For this review, take the finished solid that the model builds, in its own axes (mm). A direction names the side the tool comes from. Coordinates: 2 decimals unless noted, no trailing zeros. Loops run counter-clockwise (first coordinate to the right, second up) from the corner with the lowest first, then second, coordinate; pieces in that order, holes last. Notation, with made-up numbers: (64, 75) - (116, 75) arc R28 ccw to (116, 110) - close; hole circle Ø2 at (45.25, -2). An arc over 180 degrees is marked (long way). Use one line per item in the form item = value. Start each with the question number.
1. Add section A-A on z = 2.8. Give the boundary of the cut face in (x, y), and give its area (3 significant figures).
2. Add section D-D on y = 42.75. Give the boundary of the cut face in (x, z), and give its area (3 significant figures).
3. To check wall thickness, follow probe 1 along X at (y, z) = (33, 0.1); probe 2 along X at (y, z) = (32.5, 2.55); probe 3 along X at (y, z) = (45.5, 1.45). State the ranges of each line that lie inside material, in increasing order.
4. Draft analysis for pull direction X (two halves, no side actions). For faces 1 (the face through (98.017, 29, 2)), 2 (the face through (81, 36.5, 3.25)), 3 (the face through (83.767, 34, 2)), state which applies: +X half, -X half, draft (parallel to the pull), parting line (faces both ways), or undercut.
5. Add section C-C on x = 95.5. Give the boundary of the cut face in (y, z).
6. For pin 1 Ø1 at (x, z) = (82, 1) entering from -Y; pin 2 Ø1 at (y, z) = (46, 2.5) entering from +X; pin 3 Ø1.6 at (y, z) = (24, 1.5) entering from -X, all flat-tipped, find the tip position at first contact; note any pin that passes through.
7. Machinability: for faces 4 (the face through (66, 27.022, 2)), 5 (the face through (94.767, 34, 2)), 6 (the face through (94.767, 25, 2)), 7 (the face through (67.767, 34, 2)), which of the approach directions +Z, -Z, +X, -X, +Y, -Y give a long, thin tool a straight path to every point of the face, cutting with its end or side? Answer none if there is none.
8. Add section B-B on y = 33.25. Give the boundary of the cut face in (x, z), and give its area (3 significant figures).
Autodesk Inventor part; units mm, degrees
ref_plane "YZ Plane" through (0, 0, 0) normal (1, 0, 0) x (0, 1, 0)
ref_plane "XZ Plane" through (0, 0, 0) normal (0, 1, 0) x (-1, 0, 0)
ref_plane "XY Plane" through (0, 0, 0) normal (0, 0, 1) x (1, 0, 0)
sketch "Block1" plane through (0, 0, 0) normal (0, 0, 1) x (1, 0, 0)
  circle A0 centre (74.029, 24.2723) radius 1
  line L0 (49.279, 30.4723) -> (71.779, 30.4723)
  line L1 (71.779, 30.4723) -> (71.779, 18.0723)
  line L2 (71.779, 18.0723) -> (49.279, 18.0723)
  line L3 (49.279, 18.0723) -> (49.279, 30.4723)
  line L4 (49.279, 30.4723) -> (44.779, 30.4723)
  line L5 (44.779, 30.4723) -> (44.779, 18.0723)
  line L6 (44.779, 18.0723) -> (49.279, 18.0723)
  line L7 (49.279, 18.0723) -> (49.279, 30.4723)
  line L8 (71.779, 30.4723) -> (76.279, 30.4723)
  line L9 (76.279, 30.4723) -> (76.279, 18.0723)
  line L10 (76.279, 18.0723) -> (71.779, 18.0723)
  line L11 (71.779, 18.0723) -> (71.779, 30.4723)
  line L12 (44.779, 24.2723) -> (76.279, 24.2723) construction
  line L13 (47.029, 30.4723) -> (47.029, 18.0723) construction
  circle A1 centre (47.029, 24.2723) radius 1
  line L14 (74.029, 30.4723) -> (74.029, 18.0723) construction
  point P0 (60.979, 24.0984)
  dimension "d7" = 22.5
  dimension "d8" = 12.4
  dimension "d9" = 4.5
  dimension "d10" = 4.5
  dimension "d11" = 2
  dimension "d12" = 2
sketch "Sketch1" plane through (0, 0, 0) normal (0, 0, 1) x (1, 0, 0)
  line L0 (-92.7646, -8.503) -> (-89.7646, -8.503)
  line L1 (-89.7646, -8.503) -> (-89.7646, -11.753)
  line L2 (-89.7646, -11.753) -> (-92.7646, -11.753)
  line L3 (-92.7646, -11.753) -> (-92.7646, -8.503)
  line L4 (-92.7646, -21.6527) -> (-89.7646, -21.6527)
  line L5 (-89.7646, -21.6527) -> (-89.7646, -21.7527)
  line L6 (-89.7646, -21.7527) -> (-92.7646, -21.7527)
  line L7 (-92.7646, -21.7527) -> (-92.7646, -21.6527)
  line L8 (67.7668, 36.0225) -> (94.7668, 36.0225)
  line L9 (94.7668, 36.0225) -> (94.7668, 23.0225)
  line L10 (94.7668, 23.0225) -> (67.7668, 23.0225)
  line L11 (67.7668, 23.0225) -> (67.7668, 36.0225)
  line L12 (67.7668, 29.5225) -> (94.7668, 29.5225) construction
  line L13 (64.5168, 32.0225) -> (67.7668, 32.0225)
  line L14 (67.7668, 32.0225) -> (67.7668, 27.0225)
  line L15 (67.7668, 27.0225) -> (64.5168, 27.0225)
  line L16 (64.5168, 27.0225) -> (64.5168, 32.0225)
  line L17 (64.5168, 29.5225) -> (67.7668, 29.5225) construction
  line L18 (81.2668, 36.0225) -> (81.2668, 23.0225) construction
  line L19 (78.7668, 36.0225) -> (83.7668, 36.0225)
  line L20 (83.7668, 36.0225) -> (83.7668, 32.7725)
  line L21 (83.7668, 32.7725) -> (78.7668, 32.7725)
  line L22 (78.7668, 32.7725) -> (78.7668, 36.0225)
  line L23 (81.2668, 36.0225) -> (81.2668, 32.7725) construction
  line L24 (98.0168, 32.0225) -> (94.7668, 32.0225)
  line L25 (94.7668, 32.0225) -> (94.7668, 27.0225)
  line L26 (94.7668, 27.0225) -> (98.0168, 27.0225)
  line L27 (98.0168, 27.0225) -> (98.0168, 32.0225)
  line L28 (98.0168, 29.5225) -> (94.7668, 29.5225) construction
  line L29 (78.7668, 23.0225) -> (83.7668, 23.0225)
  line L30 (83.7668, 23.0225) -> (83.7668, 26.2725)
  line L31 (83.7668, 26.2725) -> (78.7668, 26.2725)
  line L32 (78.7668, 26.2725) -> (78.7668, 23.0225)
  line L33 (81.2668, 23.0225) -> (81.2668, 26.2725) construction
  arc A0 (94.7668, 36.0225) -> (67.7668, 36.0225) centre (81.2668, 36.0225) ccw
  point P0 (0, 0)
  dimension "d0" = 3
  dimension "mat" = 3.25
  dimension "d2" = 3
  dimension "d3" = 0.1
  dimension "d58" = 27
  dimension "d59" = 13
  dimension "d60" = 3.25
  dimension "d61" = 5
  dimension "d68" = 5
  dimension "d69" = 3.25
extrude "Extrusion5" add sketch "Sketch1" along normal blind 3.25 contours L8 L22 L21 L20 L9 L10 L30 L31 L32 L11 | L8 L20 L21 L22 | L11 L15 L16 L13 | L32 L31 L30 L10
extrude "Extrusion7" cut sketch "Sketch1" along normal blind 3.25 contours L8 L20 L21 L22
extrude "Extrusion8" cut sketch "Sketch1" along normal blind 3.25 contours L32 L31 L30 L10
extrude "Extrusion9" add sketch "Sketch1" along normal blind 3.25 contours L24 L27 L26 L9
extrude "Extrusion10" add sketch "Sketch1" along normal blind 3.25 contours A0 L8
equation "\"d60\" = mat"
equation "\"d69\" = mat"
equation "\"d62\" = mat"
equation "\"d70\" = mat"
equation "\"d72\" = mat"
equation "\"d74\" = mat"
equation "\"d76\" = mat"
properties part number "arm-servo"
Conclusion:
q1.outline = (64.52, 27.02) - (67.77, 27.02) - (67.77, 23.02) - (78.77, 23.02) - (78.77, 26.27) - (83.77, 26.27) - (83.77, 23.02) - (94.77, 23.02) - (94.77, 27.02) - (98.02, 27.02) - (98.02, 32.02) - (94.77, 32.02) - (94.77, 36.02) arc R13.5 ccw to (67.77, 36.02) - (67.77, 32.02) - (64.52, 32.02) - close; hole (78.77, 32.77) - (83.77, 32.77) - (83.77, 36.02) - (78.77, 36.02) - close
q1.area = 637 mm^2
q2.outline = (69.56, 0) - (92.97, 0) - (92.97, 3.25) - (69.56, 3.25) - close
q2.area = 76.1 mm^2
q3.probe_1 = 67.77 to 78.77, 83.77 to 94.77
q3.probe_2 = 67.77 to 94.77
q3.probe_3 = 71.65 to 90.88
q4.face_1 = +X half
q4.face_2 = draft
q4.face_3 = undercut
q5.outline = (27.02, 0) - (32.02, 0) - (32.02, 3.25) - (27.02, 3.25) - close
q6.pin_1 = 26.27
q6.pin_2 = 90.88
q6.pin_3 = 67.77
q7.face_4 = +Z, -Z, -X, -Y
q7.face_5 = +Z, -Z, +X, +Y
q7.face_6 = +Z, -Z, +X, -Y
q7.face_7 = +Z, -Z, -X, +Y
q8.outline = (67.77, 0) - (78.77, 0) - (78.77, 3.25) - (67.77, 3.25) - close; (83.77, 0) - (94.77, 0) - (94.77, 3.25) - (83.77, 3.25) - close
q8.area = 71.5 mm^2
